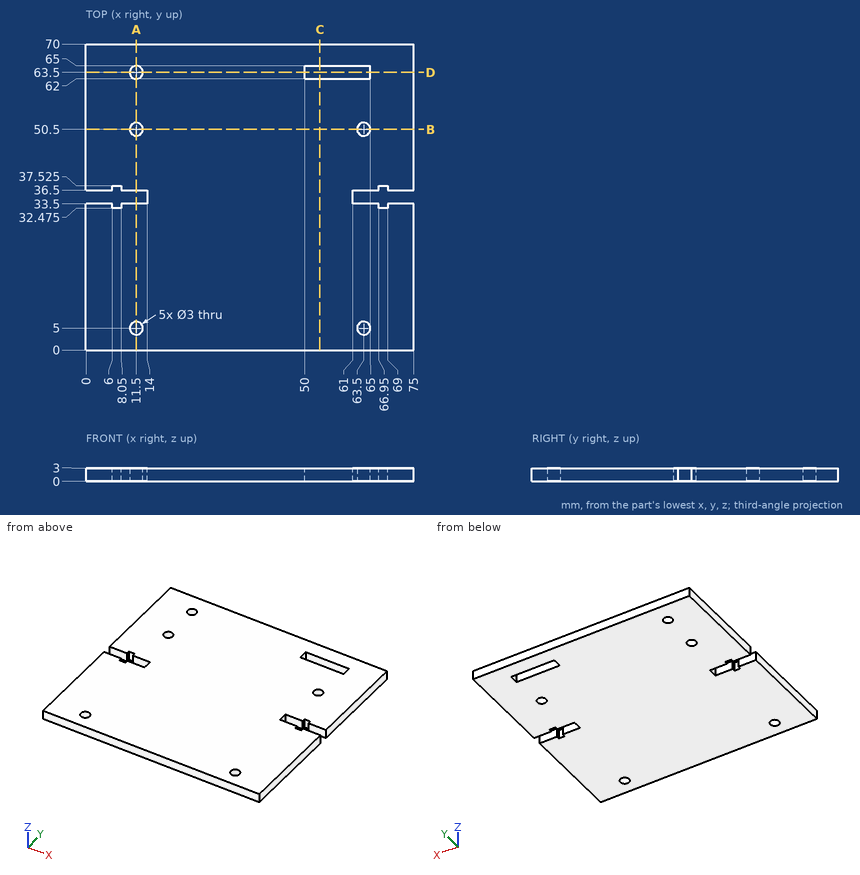
The drawing under review shows one solid part. Ordinate dimensions are in mm from its lowest x, y, z. Give positions to 0.01 mm unless a question says otherwise; leave off trailing zeros. Loops run counter-clockwise (first coordinate to the right, second up) from the corner with the lowest first, then second, coordinate; pieces in that order, holes last. Notation, with made-up numbers: M 4,87 L 16,87 A21 cw 16,116 Z; hole C -17,55 d11. An arc over 180 degrees is marked long. Return JSON: item names as keys, results as strings. Group by question number.
Item 1: Insertion check: pin 1 Ø1.8 at (x, y) = (63.5, 5) entering from +Z. The pin has a flat end and moves straight along its axis. Give the tip position at first contact, or say it passes through.
Item 2: For probe 1 along Y at (x, z) = (63.5, 0.8); probe 2 along Y at (x, z) = (64.5, 0.7); probe 3 along Y at (x, z) = (7.5, 0.9) (3 decimals), list the stretches that pass through material, from the lowest coordinate up.
Item 3: We need section C-C (x = 53.5). Give the boundary of the cut face in (y, z).
Item 4: We need section A-A (x = 11.5). Give the boundary of the cut face in (y, z), and give its area (3 significant figures).
Item 5: We need section B-B (y = 50.5). Give the boundary of the cut face in (x, z), and give its area (3 significant figures).
Item 6: We need section D-D (y = 63.5). Give the boundary of the cut face in (x, z).
Output:
{
 "1": {"pin 1": "passes through"},
 "2": {"probe 1": "y = 0 to 3.5, 6.5 to 33.5, 36.5 to 49, 52 to 62, 65 to 70", "probe 2": "y = 0 to 3.88, 6.12 to 33.5, 36.5 to 49.38, 51.62 to 62, 65 to 70", "probe 3": "y = 0 to 32.475, 37.525 to 70"},
 "3": {"outline": "M 0,0 L 62,0 L 62,3 L 0,3 Z; M 65,0 L 70,0 L 70,3 L 65,3 Z"},
 "4": {"outline": "M 0,0 L 3.5,0 L 3.5,3 L 0,3 Z; M 6.5,0 L 33.5,0 L 33.5,3 L 6.5,3 Z; M 36.5,0 L 49,0 L 49,3 L 36.5,3 Z; M 52,0 L 62,0 L 62,3 L 52,3 Z; M 65,0 L 70,0 L 70,3 L 65,3 Z", "area": "174 mm^2"},
 "5": {"outline": "M 0,0 L 10,0 L 10,3 L 0,3 Z; M 13,0 L 62,0 L 62,3 L 13,3 Z; M 65,0 L 75,0 L 75,3 L 65,3 Z", "area": "207 mm^2"},
 "6": {"outline": "M 0,0 L 10,0 L 10,3 L 0,3 Z; M 13,0 L 50,0 L 50,3 L 13,3 Z; M 65,0 L 75,0 L 75,3 L 65,3 Z"}
}
